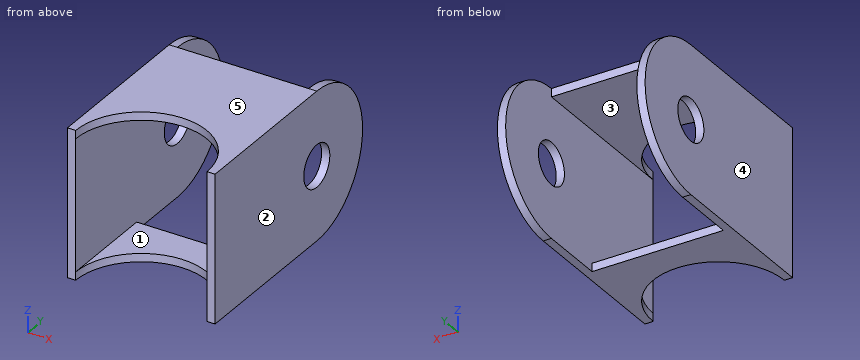
```python
from build123d import *

# Parameters (mm, degrees)
SKETCH1_W               = 28.575
SKETCH1_H               = 28.575
SKETCH1_W_2             = 25.4
SKETCH1_H_2             = 25.4
BOSS_EXTRUDE1_DEPTH     = 31.75
SKETCH2_R               = 14.2875
BOSS_EXTRUDE2_DEPTH     = 1.5875
BOSS_EXTRUDE3_START     = -1.5875
SKETCH3_R               = 14.2875
BOSS_EXTRUDE3_DEPTH     = 1.5875
CUT_EXTRUDE1_DEPTH      = 57.036726238
CUT_EXTRUDE1_DEPTH_BACK = 57.036726238
SKETCH4_R               = 4.064
CUT_EXTRUDE2_DEPTH      = 57.036726238
CUT_EXTRUDE2_DEPTH_BACK = 57.036726238
SKETCH5_R               = 12.7
CUT_EXTRUDE3_REACH      = 57.244
SKETCH6_W               = 25.4
SKETCH6_H               = 12.7


with BuildPart() as part:
    # Sketch1 → Boss-Extrude1 (new body)
    with BuildSketch(Plane(origin=(0, 0, 0), x_dir=(1, 0, 0), z_dir=(0, 1, 0))):
        Rectangle(SKETCH1_W, SKETCH1_H)
        Rectangle(SKETCH1_W_2, SKETCH1_H_2, mode=Mode.SUBTRACT)
    extrude(amount=BOSS_EXTRUDE1_DEPTH)

    # Sketch2 → Boss-Extrude2 (add)
    with BuildSketch(Plane.ZY.offset(14.2875)):
        with Locations((0, 31.75)):
            Circle(SKETCH2_R)
    extrude(amount=-BOSS_EXTRUDE2_DEPTH)

    # Sketch3 → Boss-Extrude3 (add)
    with BuildSketch(Plane(origin=(14.2875, 0, 0), x_dir=(0, 0, -1), z_dir=(1, 0, 0)).offset(BOSS_EXTRUDE3_START)):
        with Locations((0, 31.75)):
            Circle(SKETCH3_R)
    extrude(amount=BOSS_EXTRUDE3_DEPTH)

    # Sketch4 → Cut-Extrude1 (cut, two sides: drawn at the far end of the back side and taken through both)
    with BuildSketch(Plane.ZY.offset(14.2875).offset(-CUT_EXTRUDE1_DEPTH_BACK)):
        with Locations(Location((0, 31.75, 0), (0, 0, 180))):
            Circle(SKETCH4_R)
    extrude(amount=CUT_EXTRUDE1_DEPTH + CUT_EXTRUDE1_DEPTH_BACK, mode=Mode.SUBTRACT)

    # Sketch5 → Cut-Extrude2 (cut, two sides: drawn at the far end of the back side and taken through both)
    with BuildSketch(Plane.XY.offset(14.2875).offset(-CUT_EXTRUDE2_DEPTH_BACK)):
        Circle(SKETCH5_R)
    extrude(amount=CUT_EXTRUDE2_DEPTH + CUT_EXTRUDE2_DEPTH_BACK, mode=Mode.SUBTRACT)

    # Sketch6 → Cut-Extrude3 (cut, up to next)
    with BuildSketch(Plane.XY.offset(-12.7), mode=Mode.PRIVATE) as cut_extrude3_sk1:
        with Locations((0, 25.4)):
            Rectangle(SKETCH6_W, SKETCH6_H)
    cut_extrude3_tool1 = extrude(cut_extrude3_sk1.sketch, amount=-CUT_EXTRUDE3_REACH, mode=Mode.PRIVATE) & part.part
    add(cut_extrude3_tool1.solids().sort_by_distance((0, 25.4, -12.7))[0], mode=Mode.SUBTRACT)


solid = part.part
```
CAD build for the part. Positions are in the model's coordinates, mm. Face numbers are marked on the shaded views. A direction names the side the tool comes from. Coordinates: 2 decimals unless noted, no trailing zeros. Order: outer loops, then holes, each group sorted by start corner. A loop starts at its lowest first (then second) coordinate and runs counter-clockwise, first axis right, second up. Notation, with made-up numbers: M 0,-11.75 L 5,-11.75 A25 cw 5,24.25 Z; hole C -24.5,65.5 d2. An arc over 180 degrees is marked long. Write each question's results on one line, items separated by ' | '. Start each with the question number.
Q1. Cut at C-C (z = 0). List the corners of the cut face in (x, y), then the cut area to 3 significant figures.
Q2. Cut at B-B (x = 0). List the corners of the cut face in (y, z).
Q3. Cut at D-D (y = 8.5). List the corners of the cut face in (x, z).
Q4. Pull direction X, two halves, no side cores. Call the marked faces 3, 4 and 5: +X half, -X half, draft (parallel to the pull), parting line (faces both ways), or undercut.
Q5. Which spindle directions (+Z, -Z, +X, -X, +Y, -Y) get a long thin tool onto all of the face, cutting with end or side? Do the marked faces 1 and 2. Say none if no direction does.
Q6. Flat gauge pins, fed straight in: P1, Ø0.8, axis at x = -3, z = -13.5, coming from the +Y side; P2, Ø1.7, axis at x = 2, z = 13, coming from the +Y side. Where does each tip first touch, or does it go through?
Q7. Cut at A-A (y = 18). List the corners of the cut face in (x, z).
Q8. Drill centre lines: probe 1 along Y at (x, z) = (13.9, 0); probe 2 along X at (y, z) = (3.5, -10). Where is each one in solid material? Low to high. Write a range as from..to.
Found:
1) outline: M -14.29,0 L -12.7,0 L -12.7,27.69 L -14.29,27.69 Z; M -14.29,35.81 L -12.7,35.81 L -12.7,46.04 L -14.29,46.04 Z; M 12.7,0 L 14.29,0 L 14.29,27.69 L 12.7,27.69 Z; M 12.7,35.81 L 14.29,35.81 L 14.29,46.04 L 12.7,46.04 Z | area: 120 mm²
2) outline: M 12.7,-14.29 L 19.05,-14.29 L 19.05,-12.7 L 12.7,-12.7 Z; M 12.7,12.7 L 31.75,12.7 L 31.75,14.29 L 12.7,14.29 Z
3) outline: M -14.29,-14.29 L -9.44,-14.29 L -9.44,-12.7 L -12.7,-12.7 L -12.7,12.7 L -9.44,12.7 L -9.44,14.29 L -14.29,14.29 Z; M 9.44,-14.29 L 14.29,-14.29 L 14.29,14.29 L 9.44,14.29 L 9.44,12.7 L 12.7,12.7 L 12.7,-12.7 L 9.44,-12.7 Z
4) face 3: undercut | face 4: -X half | face 5: draft
5) face 1: +Y, -Y | face 2: +Z, -Z, +X, +Y, -Y
6) P1: y = 19.05 | P2: y = 31.75
7) outline: M -14.29,-14.29 L 14.29,-14.29 L 14.29,14.29 L -14.29,14.29 Z; hole M -12.7,-12.7 L 12.7,-12.7 L 12.7,12.7 L -12.7,12.7 Z
8) probe 1: 0..27.69, 35.81..46.04 | probe 2: -14.29..-12.7, 12.7..14.29
